```python
from build123d import *

# Parameters (mm, degrees)
F1_W     = 380
F1_H     = 14
F2_DEPTH = 11
F4_DEPTH = 380.001
F5_R     = 9
F6_DEPTH = 22
F8_R     = 3
F7_W     = 380
F7_H     = 22
F9_DEPTH = 0.7
F10_R    = 1


with BuildPart() as f2:
    # F1 (on Front) → F2 (new body, symmetric)
    with BuildSketch(Plane.XZ):
        with Locations((0, 7)):
            Rectangle(F1_W, F1_H)
    extrude(amount=F2_DEPTH, both=True)

    # F3 (on face) → F4 (cut, through all)
    with BuildSketch(Plane(origin=(-190, 0, 0), x_dir=(0, -1, 0), z_dir=(-1, 0, 0))):
        with BuildLine():
            Line((7.6, 14), (-7.6, 14))
            Line((-7.6, 14), (-7.6, 5.4))
            ThreePointArc((-7.6, 5.4), (-7.0142135624, 3.9857864376), (-5.6, 3.4))
            Line((-5.6, 3.4), (5.6, 3.4))
            ThreePointArc((5.6, 3.4), (7.0142135624, 3.9857864376), (7.6, 5.4))
            Line((7.6, 5.4), (7.6, 14))
        make_face()
    extrude(amount=-F4_DEPTH, mode=Mode.SUBTRACT)

    # F5 (on face) → F6 (join, through all)
    with BuildSketch(Plane(origin=(0, 11, 0), x_dir=(-1, 0, 0), z_dir=(0, 1, 0))):
        with BuildLine():
            Line((-9.7979589711, 0), (-72, 0))
            Line((-72, 0), (-13.9642400438, -9))
            ThreePointArc((-13.9642400438, -9), (-12.7047442125, -4.118718295), (-9.7979589711, 0))
        make_face()
        with BuildLine():
            ThreePointArc((-9.7979589711, 0), (-12.7047442125, -4.118718295), (-13.9642400438, -9))
            ThreePointArc((-13.9642400438, -9), (-0.5003195915, -23.9910571547), (14, -10))
            ThreePointArc((14, -10), (13.9910571547, -9.4996804085), (13.9642400438, -9))
            ThreePointArc((13.9642400438, -9), (12.7047442125, -4.118718295), (9.7979589711, 0))
            Line((9.7979589711, 0), (-9.7979589711, 0))
        make_face()
        with Locations((0, -10)):
            Circle(F5_R, mode=Mode.SUBTRACT)
        with BuildLine():
            Line((72, 0), (9.7979589711, 0))
            ThreePointArc((9.7979589711, 0), (12.7047442125, -4.118718295), (13.9642400438, -9))
            Line((13.9642400438, -9), (72, 0))
        make_face()
    extrude(amount=-F6_DEPTH)

    # F8
    f8_edges = [f2.edges().sort_by_distance(p)[0] for p in [
        (190, -9.3, 14),
        (190, 9.3, 14),
        (190, 0, 0),
        (-190, -9.3, 14),
        (-190, 9.3, 14),
        (-190, 0, 0),
        (13.96424, 0, -9),
        (-13.96424, 0, -9),
    ]]
    fillet(f8_edges, radius=F8_R)

    # F7 (on face) → F9 (join)
    with BuildSketch(Plane.XY.offset(14)):
        Rectangle(F7_W, F7_H)
    extrude(amount=F9_DEPTH)

    # F10
    f10_edges = [f2.edges().sort_by_distance(p)[0] for p in [
        (-9, 0, -10),
        (9, 11, -10),
        (9, -11, -10),
    ]]
    fillet(f10_edges, radius=F10_R)


solid = f2.part
```
Geometry: final body of the model. Coordinates: model frame, mm. A direction names the side the tool comes from. Coordinates: 2 decimals unless noted, no trailing zeros. Order: outer loops, then holes, each group sorted by start corner. A loop starts at its lowest first (then second) coordinate and runs counter-clockwise, first axis right, second up. Notation, with made-up numbers: (-27.75, -21) -> (20.25, -21) arc R14 ccw to (20.25, -10) -> close; hole circle Ø5 at (19.25, 26.5). An arc over 180 degrees is marked (long way). Answer in a Markdown table with one row per item.
Item 1: Section D-D on x = 57. Output: boundary loops of the cut face in (y, z), plus the area to 3 significant figures.
Return value:
| item | result |
|---|---|
| outline | (-11, -2.33) -> (11, -2.33) -> (11, 14.7) -> (-11, 14.7) -> close; hole (-7.6, 5.4) arc R2 ccw to (-5.6, 3.4) -> (5.6, 3.4) arc R2 ccw to (7.6, 5.4) -> (7.6, 14) -> (-7.6, 14) -> close |
| area | 215 mm² |
Item 2: Section C-C on y = 0. State how many separate pieces and enclosed holes the cut face has, plus the area to 3 significant figures.
Return value:
| item | result |
|---|---|
| separate pieces | 2 |
| enclosed holes | 1 |
| area | 2,410 mm² |
Item 3: Contact query for flat-ended pins moving along their axis: P1, Ø6.5, axis at x = -18.5, y = -5, coming from the -Z side; P2, Ø11, axis at x = 157.5, y = 2.5, coming from the -Z side; P3, Ø5, axis at y = 3, z = -19.5, coming from the +X side. Output: stop coordinate, or through.
Return value:
| item | result |
|---|---|
| P1 | stops at z = -9.09 |
| P2 | stops at z = 0 |
| P3 | stops at x = 12.12 |
Item 4: Section A-A on x = 0. Output: boundary loops of the cut face in (y, z).
Return value:
| item | result |
|---|---|
| outline | (-11, -24) -> (11, -24) -> (11, -20) arc R1 ccw to (10, -19) -> (-10, -19) arc R1 ccw to (-11, -20) -> close; (-11, 0) arc R1 ccw to (-10, -1) -> (10, -1) arc R1 ccw to (11, 0) -> (11, 14.7) -> (-11, 14.7) -> close; hole (-7.6, 5.4) arc R2 ccw to (-5.6, 3.4) -> (5.6, 3.4) arc R2 ccw to (7.6, 5.4) -> (7.6, 14) -> (-7.6, 14) -> close |
Item 5: Ray query, L1, parallel to Z at x = 0, y = -3; L2, parallel to Z at x = 175, y = 2.5; L3, parallel to Y at x = 131.5, z = 5. Return the intervals inside material, ascending.
Return value:
| item | result |
|---|---|
| L1 | z = -24 to -19, -1 to 3.4, 14 to 14.7 |
| L2 | z = 0 to 3.4, 14 to 14.7 |
| L3 | y = -11 to -7.56, 7.56 to 11 |
Item 6: Draft query along X for faces 5 (the flat face through (190, 6.5, 3.4)), 6 (the cylindrical face through (1.951, 0.14, -18.786)), 7 (the flat face through (-3, 7.6, 10)). Return one class per face: released by +X, released by -X, zero draft, split by the parting line, or undercut.
Return value:
| item | result |
|---|---|
| face 5 | released by +X |
| face 6 | undercut |
| face 7 | zero draft |
Item 7: Access query for faces 1 (the flat face through (129, 0, 0)), 2 (the flat face through (-130, 0, 0)), 3 (the flat face through (-3, -7.6, 10)), 4 (the flat face through (-3, 11, 8)). Directions: +Z, -Z, +X, -X, +Y, -Y. A direction counts if a zero-diameter tool reaches every point of the face in a straight line with its end or side. Return the directions, or none.
Return value:
| item | result |
|---|---|
| face 1 | -Z, +X, +Y, -Y |
| face 2 | -Z, -X, +Y, -Y |
| face 3 | +X, -X |
| face 4 | +Z, -Z, +X, -X, +Y |
Item 8: Section B-B on x = -145.5. Output: boundary loops of the cut face in (y, z).
Return value:
| item | result |
|---|---|
| outline | (-11, 0) -> (11, 0) -> (11, 14.7) -> (-11, 14.7) -> close; hole (-7.6, 5.4) arc R2 ccw to (-5.6, 3.4) -> (5.6, 3.4) arc R2 ccw to (7.6, 5.4) -> (7.6, 14) -> (-7.6, 14) -> close |
